Work out the finished part from the listing and answer in its coordinate system (mm). A direction names the side the tool comes from. Give positions to 0.01 mm unless a question says otherwise; leave off trailing zeros. Order: outer loops, then holes, each group sorted by start corner. A loop starts at its lowest first (then second) coordinate and runs counter-clockwise, first axis right, second up.
Autodesk Inventor part; units mm, degrees
ref_plane "YZ Plane" through (0, 0, 0) normal (1, 0, 0) x (0, 1, 0)
ref_plane "XZ Plane" through (0, 0, 0) normal (0, 1, 0) x (-1, 0, 0)
ref_plane "XY Plane" through (0, 0, 0) normal (0, 0, 1) x (1, 0, 0)
sketch "스케치1" plane through (0, 0, 0) normal (0, 0, 1) x (1, 0, 0)
  circle A0 centre (0, 0) radius 29
  circle A1 centre (-24.5, 0) radius 1.5
  circle A2 centre (-24.5, 0) radius 2.75
  circle A3 centre (0, -24.5) radius 1.5
  circle A4 centre (0, -24.5) radius 2.75
  circle A5 centre (24.5, 0) radius 1.5
  circle A6 centre (24.5, 0) radius 2.75
  circle A7 centre (0, 24.5) radius 1.5
  circle A8 centre (0, 24.5) radius 2.75
  dimension "d0" = 58
  dimension "d1" = 3
  dimension "d2" = 5.5
  dimension "d3" = 24.5
  dimension "d6" = 360
extrude "돌출1" add sketch "스케치1" along normal blind 6 contours A0 | A2 | A4 | A6 | A8
sketch "스케치2" plane through (0, 0, 6) normal (0, 0, 1) x (1, 0, 0)
  circle A0 centre (0, 24.5) radius 1.5
  circle A1 centre (24.5, 0) radius 1.5
  circle A2 centre (0, -24.5) radius 1.5
  circle A3 centre (-24.5, 0) radius 1.5
  circle A4 centre (-24.5, 0) radius 2.75
  circle A5 centre (24.5, 0) radius 2.75
  circle A6 centre (0, -24.5) radius 2.75
  circle A7 centre (0, 24.5) radius 2.75
extrude "돌출2" cut sketch "스케치2" against normal blind 4
sketch "스케치5" plane through (0, 0, 0) normal (0, 0, -1) x (-1, 0, 0)
  circle A0 centre (0, 0) radius 65
  circle A1 centre (7.157, 23.4313) radius 1
  line L0 (22.2881, 36.3872) -> (18.0584, 32.156)
  arc A2 (18.0584, 32.156) -> (18.0588, 29.3276) centre (19.4728, 30.742) ccw
  line L1 (18.0588, 29.3276) -> (29.3745, 18.0158)
  arc A3 (29.3745, 18.0158) -> (32.2029, 18.0163) centre (30.7884, 19.4302) ccw
  line L2 (32.2029, 18.0163) -> (36.4326, 22.2474)
  arc A4 (36.4326, 22.2474) -> (36.4322, 25.0758) centre (35.0182, 23.6614) ccw
  line L3 (36.4322, 25.0758) -> (25.1165, 36.3876)
  arc A5 (25.1165, 36.3876) -> (22.2881, 36.3872) centre (23.7025, 34.9732) ccw
  circle A6 centre (0, 24.5) radius 1.2295
  circle A7 centre (-24.5, 0) radius 1.2295
  circle A8 centre (0, -24.5) radius 1.2295
  circle A9 centre (24.5, 0) radius 1.2295
  circle A10 centre (0, 51.0531) radius 2.5
  circle A11 centre (0, -51.0531) radius 2.5
  circle A12 centre (-51.0531, 0) radius 2.5
  circle A13 centre (51.0531, 0) radius 2.5
  circle A14 centre (-22.9994, -55.4169) radius 1.5
  circle A15 centre (55.4169, -22.9994) radius 1.5
  circle A16 centre (22.9994, 55.4169) radius 1.5
  circle A17 centre (-55.4169, 22.9994) radius 1.5
  circle A18 centre (-22.9226, 55.4487) radius 1.5
  circle A19 centre (55.4487, 22.9226) radius 1.5
  circle A20 centre (22.9226, -55.4487) radius 1.5
  circle A21 centre (-55.4487, -22.9226) radius 1.5
  circle A22 centre (0, 0) radius 65
  circle A23 centre (0, 0) radius 25
  line L4 (-20.0138, -19.9861) -> (19.9861, -20.0138)
  line L5 (19.9861, -20.0138) -> (20.0138, 19.9861)
  line L6 (20.0138, 19.9861) -> (-19.9861, 20.0138)
  line L7 (-19.9861, 20.0138) -> (-20.0138, -19.9861)
  circle A24 centre (24.3126, 5.8222) radius 1
  dimension "d14" = 50
  dimension "d15" = 2
extrude "돌출3" cut sketch "스케치5" against normal blind 3 contours A24 A23 | A23 A24
properties part number "접촉부 철판가공"
1. The part is cut by section B-B (x = 24.5). Write down the section's boundary in (y, z).
Findings below:
outline: (-15.52, 0) - (-1.5, 0) - (-1.5, 2) - (-2.75, 2) - (-2.75, 6) - (-15.52, 6) - close; (1.5, 0) - (15.52, 0) - (15.52, 6) - (2.75, 6) - (2.75, 2) - (1.5, 2) - close
2. The mould has two halves that part along Y. Classify faces 1 (the face through (0, 0, 0)), 2 (the face through (1, 23, 2)), 3 (the face through (13.38, 25.73, 2.96)): pulls with the +Y half, pulls with the -Y half, needs draft (parallel to the pull), parting line crosses it, or undercut.
Findings below:
face 1: needs draft
face 2: undercut
face 3: parting line crosses it
3. Given P1, Ø2, axis at x = -25, y = 5.5, coming from the -Z side; P2, Ø3, axis at x = 1, y = -24.5, coming from the +Z side; P3, Ø2.5, axis at x = 0, y = 24.5, coming from the +Z side; P4, Ø2, axis at y = -6, z = 1, coming from the +X side, each flat-ended and moving along its own axis, determine where each tip first touches the part or whether it passes through.
Findings below:
P1: stops at z = 0
P2: stops at z = 2
P3: passes through
P4: stops at x = 28.57
4. The part is cut by section A-A (y = 0). Write down the section's boundary in (x, z).
Findings below:
outline: (-29, 0) - (-26, 0) - (-26, 2) - (-27.25, 2) - (-27.25, 6) - (-29, 6) - close; (-23, 0) - (23, 0) - (23, 2) - (21.75, 2) - (21.75, 6) - (-21.75, 6) - (-21.75, 2) - (-23, 2) - close; (26, 0) - (29, 0) - (29, 6) - (27.25, 6) - (27.25, 2) - (26, 2) - close
5. Straight lines are drawn through the part: probe 1 along Y at (x, z) = (-24.5, 2.9); probe 2 along Y at (x, z) = (-25.5, 1.9); probe 3 along X at (y, z) = (2, 4.9). For each, find the intervals that lie inside material, in ascending order.
Findings below:
probe 1: y = -15.52 to -2.75, 2.75 to 4.84, 6.8 to 15.52
probe 2: y = -13.81 to -1.12, 1.12 to 13.81
probe 3: x = -28.93 to -26.39, -22.61 to 22.61, 26.39 to 28.93
6. Which of the six approach directions +Z, -Z, +X, -X, +Y, -Y give full straight-line access (tool end or side, diameter ignored) to faces 4 (the face through (-24, 6, 3)), 5 (the face through (-0.358, 27.227, 4.028)), 6 (the face through (0, 23, 1))?
Findings below:
face 4: -Z
face 5: +Z
face 6: +Z, -Z
7. The part is cut by section D-D (z = 5.3). Write down the section's boundary in (x, y).
Findings below:
outline: circle Ø58 at (0, 0); hole circle Ø5.5 at (-24.5, 0); hole circle Ø5.5 at (0, -24.5); hole circle Ø5.5 at (0, 24.5); hole circle Ø5.5 at (24.5, 0)
